Part model, mm, in its own coordinate system. Face numbers are marked on the shaded views. A direction names the side the tool comes from. Coordinates: 2 decimals unless noted, no trailing zeros. Order: outer loops, then holes, each group sorted by start corner. A loop starts at its lowest first (then second) coordinate and runs counter-clockwise, first axis right, second up. Notation, with made-up numbers: (64.25, 41) - (106.25, 41) arc R18 cw to (106.25, 75) - close; hole circle Ø11 at (1.5, -37). An arc over 180 degrees is marked (long way). Use a Markdown table: item, result. Add a question column.
1) Tool access for the marked faces 4 and 5: list every direction of +Z, -Z, +X, -X, +Y, -Y with a clear straight run to the whole face (end or side of a thin tool).
2) Saw through at C-C on y = 17.5. List the corners of the cut face in (x, z).
3) Saw through at A-A on x = 25. List the corners of the cut face in (y, z), then the cut area to 4 significant figures.
4) Saw through at B-B on z = -12. List the corners of the cut face in (x, y), then the cut area to 3 significant figures.
5) Wall check: L1, parallel to Y at x = 25, z = 5.25; L2, parallel to Z at x = 12, y = 8; L3, parallel to X at y = 16, z = 4. Give the ranges that are in metal, low to high. Write a range as [from, to].
6) Saw through at D-D on y = 4. List the corners of the cut face in (x, z), then the cut area to 3 significant figures.
7) Two-plate mould, pull along X, no slides. Class the marked faces 1, 2 and 3: +X half, -X half, draft (parallel to the pull), parting line (faces both ways), or undercut.
8) Drop flat-ended pins along their axis: P1, Ø12, axis at x = 43, y = 36, coming from the -Z side; P2, Ø4, axis at x = 32.5, z = -10.5, coming from the +Y side; P3, Ø2, axis at x = 5, z = -2, coming from the -Y side. Give the stop position or say it passes through.
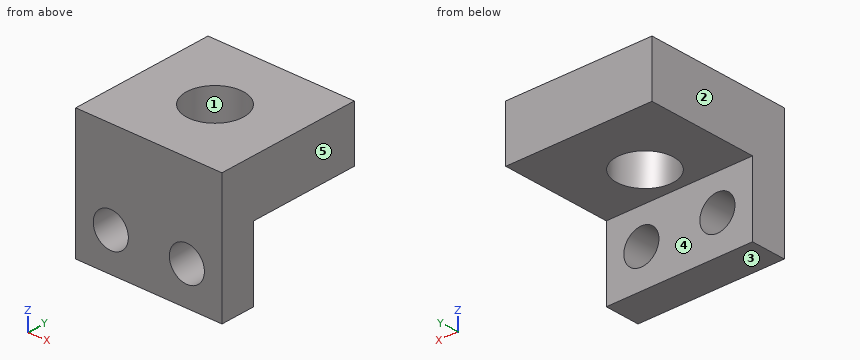
```python
from build123d import *

# Parameters (mm, degrees)
F0_W     = 50
F0_H     = 50
F0_R     = 9.75
F1_DEPTH = 19
F2_W     = 50
F2_H     = 12
F3_DEPTH = 25
F4_R     = 6
F5_DEPTH = 12.001


with BuildPart() as f1:
    # F0 (on Top) → F1 (new body)
    with BuildSketch(Plane.XY):
        with Locations((25, 25)):
            Rectangle(F0_W, F0_H)
        with Locations((25, 25)):
            Circle(F0_R, mode=Mode.SUBTRACT)
    extrude(amount=F1_DEPTH)

    # F2 (on face) → F3 (join)
    with BuildSketch(Plane(origin=(0, 0, 0), x_dir=(1, 0, 0), z_dir=(0, 0, -1))):
        with Locations((25, -6)):
            Rectangle(F2_W, F2_H)
    extrude(amount=F3_DEPTH)

    # F4 (on face) → F5 (cut, through all)
    with BuildSketch(Plane(origin=(0, 12, 0), x_dir=(-1, 0, 0), z_dir=(0, 1, 0))):
        with Locations((-38, -12)):
            Circle(F4_R)
        with Locations((-12, -12)):
            Circle(F4_R)
    extrude(amount=-F5_DEPTH, mode=Mode.SUBTRACT)


solid = f1.part
```
Results are:
| question | item | result |
|---|---|---|
| 1 | face 4 | -Z, +X, -X, +Y |
| 1 | face 5 | +Z, -Z, +X, +Y, -Y |
| 2 | outline | (0, 0) - (18.77, 0) - (18.77, 19) - (0, 19) - close; (31.23, 0) - (50, 0) - (50, 19) - (31.23, 19) - close |
| 3 | outline | (0, -25) - (12, -25) - (12, 0) - (15.25, 0) - (15.25, 19) - (0, 19) - close; (34.75, 0) - (50, 0) - (50, 19) - (34.75, 19) - close |
| 3 | area | 879.5 mm2 |
| 4 | outline | (0, 0) - (6, 0) - (6, 12) - (0, 12) - close; (18, 0) - (32, 0) - (32, 12) - (18, 12) - close; (44, 0) - (50, 0) - (50, 12) - (44, 12) - close |
| 4 | area | 312 mm2 |
| 5 | L1 | [0, 15.25], [34.75, 50] |
| 5 | L2 | [-25, -18], [-6, 19] |
| 5 | L3 | [0, 21.25], [28.75, 50] |
| 6 | outline | (0, -25) - (50, -25) - (50, 19) - (0, 19) - close; hole circle Ø12 at (12, -12); hole circle Ø12 at (38, -12) |
| 6 | area | 1,970 mm2 |
| 7 | face 1 | undercut |
| 7 | face 2 | -X half |
| 7 | face 3 | draft |
| 8 | P1 | z = 0 |
| 8 | P2 | y = 12 |
| 8 | P3 | y = 0 |
